```python
from build123d import *

# Parameters (mm, degrees)
SKETCH1_W           = 152.4
SKETCH1_H           = 241.3
BOSS_EXTRUDE1_DEPTH = 3.175
SKETCH2_W           = 3.429
SKETCH2_H           = 168.148
SKETCH2_H_2         = 40.386
CUT_EXTRUDE1_DEPTH  = 286.414664348
SKETCH3_W           = 119.38
SKETCH3_H           = 119.38
SKETCH3_W_2         = 74.6125
SKETCH3_H_2         = 25.4
SKETCH3_W_3         = 12.7
SKETCH3_H_3         = 16.256
SKETCH3_W_4         = 5.334
SKETCH3_H_4         = 7.239
CUT_EXTRUDE2_DEPTH  = 286.414664348
SKETCH4_W           = 194.284224207
SKETCH4_H           = 180.265938869
CUT_EXTRUDE4_DEPTH  = 286.414664348


with BuildPart() as part:
    # Sketch1 → Boss-Extrude1 (new body)
    with BuildSketch(Plane.XY):
        with Locations((76.2, 120.65)):
            Rectangle(SKETCH1_W, SKETCH1_H)
    extrude(amount=BOSS_EXTRUDE1_DEPTH)

    # Sketch2 → Cut-Extrude1 (cut, through all)
    with BuildSketch(Plane.XY.offset(3.175)):
        with Locations((150.6855, 139.065)):
            Rectangle(SKETCH2_W, SKETCH2_H)
        with Locations((1.7145, 139.065)):
            Rectangle(SKETCH2_W, SKETCH2_H)
        with Locations((150.6855, 20.193)):
            Rectangle(SKETCH2_W, SKETCH2_H_2)
        with Locations((1.7145, 20.193)):
            Rectangle(SKETCH2_W, SKETCH2_H_2)
    extrude(amount=-CUT_EXTRUDE1_DEPTH, mode=Mode.SUBTRACT)

    # Sketch3 → Cut-Extrude2 (cut, through all)
    with BuildSketch(Plane.XY.offset(3.175)):
        Polygon((128.016, 57.15), (140.716, 57.15), (140.716, 44.45), align=None)
        Polygon((125.77093597, 42.20493597), (138.47093597, 42.20493597), (125.77093597, 54.90493597), align=None)
        Polygon((108.966, 57.15), (121.666, 57.15), (121.666, 44.45), align=None)
        Polygon((119.42093597, 42.20493597), (106.72093597, 54.90493597), (106.72093597, 42.20493597), align=None)
        Polygon((89.916, 57.15), (102.616, 57.15), (102.616, 44.45), align=None)
        Polygon((100.37093597, 42.20493597), (87.67093597, 54.90493597), (87.67093597, 42.20493597), align=None)
        Polygon((70.866, 57.15), (83.566, 57.15), (83.566, 44.45), align=None)
        Polygon((81.32093597, 42.20493597), (68.62093597, 54.90493597), (68.62093597, 42.20493597), align=None)
        Polygon((51.816, 57.15), (64.516, 57.15), (64.516, 44.45), align=None)
        Polygon((62.27093597, 42.20493597), (49.57093597, 54.90493597), (49.57093597, 42.20493597), align=None)
        Polygon((32.766, 57.15), (45.466, 57.15), (45.466, 44.45), align=None)
        Polygon((43.22093597, 42.20493597), (30.52093597, 54.90493597), (30.52093597, 42.20493597), align=None)
        Polygon((13.716, 57.15), (26.416, 57.15), (26.416, 44.45), align=None)
        Polygon((24.17093597, 42.20493597), (11.47093597, 54.90493597), (11.47093597, 42.20493597), align=None)
        Polygon((128.016, 38.1), (140.716, 38.1), (140.716, 25.4), align=None)
        with Locations((76.454, 129.159)):
            Rectangle(SKETCH3_W, SKETCH3_H)
        Polygon((125.77093597, 23.15493597), (138.47093597, 23.15493597), (125.77093597, 35.85493597), align=None)
        Polygon((108.966, 38.1), (121.666, 38.1), (121.666, 25.4), align=None)
        Polygon((119.42093597, 23.15493597), (106.72093597, 35.85493597), (106.72093597, 23.15493597), align=None)
        Polygon((89.916, 38.1), (102.616, 38.1), (102.616, 25.4), align=None)
        Polygon((100.37093597, 23.15493597), (87.67093597, 35.85493597), (87.67093597, 23.15493597), align=None)
        Polygon((70.866, 38.1), (83.566, 38.1), (83.566, 25.4), align=None)
        Polygon((81.32093597, 23.15493597), (68.62093597, 35.85493597), (68.62093597, 23.15493597), align=None)
        Polygon((51.816, 38.1), (64.516, 38.1), (64.516, 25.4), align=None)
        Polygon((62.27093597, 23.15493597), (49.57093597, 35.85493597), (49.57093597, 23.15493597), align=None)
        Polygon((32.766, 38.1), (45.466, 38.1), (45.466, 25.4), align=None)
        Polygon((43.22093597, 23.15493597), (30.52093597, 35.85493597), (30.52093597, 23.15493597), align=None)
        Polygon((13.716, 38.1), (26.416, 38.1), (26.416, 25.4), align=None)
        Polygon((24.17093597, 23.15493597), (11.47093597, 35.85493597), (11.47093597, 23.15493597), align=None)
        Polygon((128.016, 19.05), (140.716, 19.05), (140.716, 6.35), align=None)
        Polygon((125.77093597, 4.10493597), (138.47093597, 4.10493597), (125.77093597, 16.80493597), align=None)
        Polygon((108.966, 19.05), (121.666, 19.05), (121.666, 6.35), align=None)
        Polygon((119.42093597, 4.10493597), (106.72093597, 16.80493597), (106.72093597, 4.10493597), align=None)
        Polygon((89.916, 19.05), (102.616, 19.05), (102.616, 6.35), align=None)
        Polygon((100.37093597, 4.10493597), (87.67093597, 16.80493597), (87.67093597, 4.10493597), align=None)
        Polygon((70.866, 19.05), (83.566, 19.05), (83.566, 6.35), align=None)
        Polygon((81.32093597, 4.10493597), (68.62093597, 16.80493597), (68.62093597, 4.10493597), align=None)
        Polygon((51.816, 19.05), (64.516, 19.05), (64.516, 6.35), align=None)
        Polygon((62.27093597, 4.10493597), (49.57093597, 16.80493597), (49.57093597, 4.10493597), align=None)
        Polygon((32.766, 19.05), (45.466, 19.05), (45.466, 6.35), align=None)
        Polygon((43.22093597, 4.10493597), (30.52093597, 16.80493597), (30.52093597, 4.10493597), align=None)
        Polygon((13.716, 19.05), (26.416, 19.05), (26.416, 6.35), align=None)
        Polygon((24.17093597, 4.10493597), (11.47093597, 16.80493597), (11.47093597, 4.10493597), align=None)
        with Locations((54.07025, 215.519)):
            Rectangle(SKETCH3_W_2, SKETCH3_H_2)
        with Locations((129.794, 210.947)):
            Rectangle(SKETCH3_W_3, SKETCH3_H_3)
        with Locations((104.0765, 206.4385)):
            Rectangle(SKETCH3_W_4, SKETCH3_H_4)
    extrude(amount=-CUT_EXTRUDE2_DEPTH, mode=Mode.SUBTRACT)

    # Sketch4 → Cut-Extrude4 (cut, through all)
    with BuildSketch(Plane.XY.offset(3.175)):
        with Locations((76.027835775, 153.632969435)):
            Rectangle(SKETCH4_W, SKETCH4_H)
    extrude(amount=-CUT_EXTRUDE4_DEPTH, mode=Mode.SUBTRACT)


solid = part.part
```
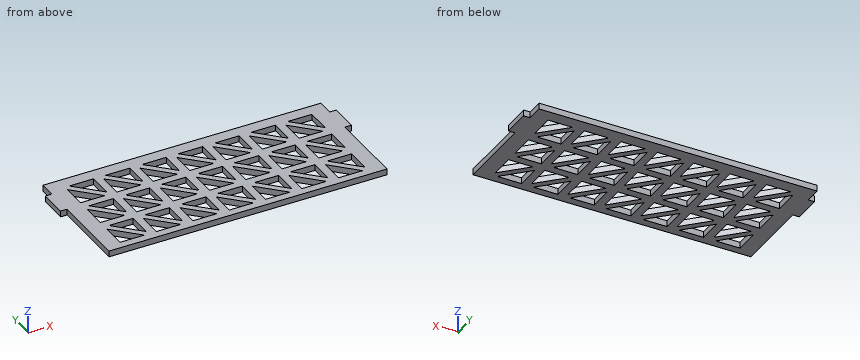
Read the model definition and answer for the solid it produces. Units are mm, in the model's axes. Give positions to 0.01 mm unless a question says otherwise; leave off trailing zeros. Order: outer loops, then holes, each group sorted by start corner. A loop starts at its lowest first (then second) coordinate and runs counter-clockwise, first axis right, second up.
(1) Find section A-A (x = 73). Give the vertices of the cut face in (y, z) (3 decimals).
(2) Find section D-D (y = 21.5). Give the vertices of the cut face in (x, z) (3 decimals), plus the area to 3 significant figures.
(3) Straight lines are drawn through the part: L1, parallel to Y at x = 120, z = 2.3; L2, parallel to Y at x = 12, z = 1.35; L3, parallel to X at y = 59, z = 1.15. For each, find the intervals that lie inside material, in ascending order.
(4) Find section B-B (y = 52). Give the number of separate pieces and of enclosed holes in the cut face, plus the area to 3 significant figures.
(5) Given pin 1 (1 mm diameter, centred on y = 48, z = 1, fed in from -X); pin 2 (1.6 mm diameter, centred on y = 29, z = 2, fed in from -X); pin 3 (1 mm diameter, centred on y = 12, z = 1.5, fed in from +X); pin 4 (1.6 mm diameter, centred on x = 2, z = 2.5, fed in from -Y), each flat-ended and moving along its own axis, determine where each tip first touches the part or whether it passes through.
Result sheet:
1. outline: (0, 0) - (4.105, 0) - (4.105, 3.175) - (0, 3.175) - close; (12.426, 0) - (16.916, 0) - (16.916, 3.175) - (12.426, 3.175) - close; (19.05, 0) - (23.155, 0) - (23.155, 3.175) - (19.05, 3.175) - close; (31.476, 0) - (35.966, 0) - (35.966, 3.175) - (31.476, 3.175) - close; (38.1, 0) - (42.205, 0) - (42.205, 3.175) - (38.1, 3.175) - close; (50.526, 0) - (55.016, 0) - (55.016, 3.175) - (50.526, 3.175) - close; (57.15, 0) - (63.5, 0) - (63.5, 3.175) - (57.15, 3.175) - close
2. outline: (3.429, 0) - (148.971, 0) - (148.971, 3.175) - (3.429, 3.175) - close
2. area: 462 mm2
3. L1: y = 0 to 8.02, 19.05 to 27.07, 38.1 to 46.12, 57.15 to 63.5
3. L2: y = 0 to 4.1, 16.28 to 23.15, 35.33 to 42.2, 54.38 to 63.5
3. L3: x = 3.43 to 148.97
4. separate pieces: 15
4. enclosed holes: 0
4. area: 252 mm2
5. pin 1: stops at x = 0
5. pin 2: stops at x = 3.43
5. pin 3: stops at x = 148.97
5. pin 4: stops at y = 40.39
